For this review, take the finished solid that the model builds, in its own axes (mm). Face numbers are marked on the shaded views. A direction names the side the tool comes from. Give positions to 0.01 mm unless a question says otherwise; leave off trailing zeros. Order: outer loops, then holes, each group sorted by start corner. A loop starts at its lowest first (then second) coordinate and runs counter-clockwise, first axis right, second up. Notation, with made-up numbers: (-2, 23.25) -> (34, 23.25) arc R27 ccw to (34, 59.25) -> close; hole circle Ø6 at (66, 46). An arc over 180 degrees is marked (long way). Use CSV: the item, a comma, the result in double quotes. Start each with the question number.
Autodesk Inventor part; units mm, degrees
ref_plane "Work Plane1" through (12.15, 0, 0) normal (1, 0, 0) x (0, 0, -1)
ref_plane "YZ Plane" through (0, 0, 0) normal (1, 0, 0) x (0, 1, 0)
ref_plane "XZ Plane" through (0, 0, 0) normal (0, 1, 0) x (-1, 0, 0)
sketch "Sketch1" plane through (0, 0, 0) normal (1, 0, 0) x (0, 1, 0)
  line L0 (0, 0) -> (7.5, 0)
  line L1 (7.5, 0) -> (3.75, -6.4952)
  line L2 (3.75, -6.4952) -> (-3.75, -6.4952)
  line L3 (-3.75, -6.4952) -> (-7.5, 0)
  line L4 (-7.5, 0) -> (-3.75, 6.4952)
  line L5 (-3.75, 6.4952) -> (3.75, 6.4952)
  line L6 (3.75, 6.4952) -> (7.5, 0)
  circle A0 centre (0, 0) radius 15
  dimension "d0" = 7.5
  dimension "d1" = 30
extrude "Extrusion1" add sketch "Sketch1" along normal blind 10.25
sketch "Sketch2" plane through (10.25, 0, 0) normal (1, 0, 0) x (0, 0, -1)
  circle A0 centre (0, 0) radius 22.5
  line L0 (-6.4952, 3.75) -> (0, 7.5)
  line L1 (-6.4952, -3.75) -> (-6.4952, 3.75)
  line L2 (0, -7.5) -> (-6.4952, -3.75)
  line L3 (6.4952, -3.75) -> (0, -7.5)
  line L4 (6.4952, 3.75) -> (6.4952, -3.75)
  line L5 (0, 7.5) -> (6.4952, 3.75)
  dimension "d4" = 45
extrude "Extrusion2" add sketch "Sketch2" against normal blind 5
sketch "Sketch3" plane through (10.25, 0, 0) normal (1, 0, 0) x (0, 0, -1)
  circle A0 centre (0, 19.05) radius 1.45
  circle A1 centre (-16.4978, -9.525) radius 1.45
  circle A2 centre (16.4978, -9.525) radius 1.45
  point P0 (0, 0)
  dimension "d11" = 360
extrude "Extrusion3" cut sketch "Sketch3" against normal up to surface (5 mm away)
sketch "Sketch4" plane through (10.25, 0, 0) normal (1, 0, 0) x (0, 0, -1)
  circle A0 centre (0, 19.05) radius 1.45
  line L0 (-3, 17.2409) -> (-3, 16.225)
  line L1 (3, 17.2409) -> (3, 16.225)
  line L2 (13.3804, 11.279) -> (12.7273, 10.5007)
  line L3 (8.7841, 15.1357) -> (8.1311, 14.3574)
  line L4 (17.5, 0.0394) -> (16.4994, -0.137)
  line L5 (16.4581, 5.9483) -> (15.4575, 5.7719)
  line L6 (13.4311, -11.2185) -> (12.5512, -10.7106)
  line L7 (16.4311, -6.0224) -> (15.5512, -5.5144)
  arc A1 (8.7841, 15.1357) -> (3, 17.2409) centre (0, 0) ccw
  arc A2 (16.4311, -6.0224) -> (17.5, 0.0394) centre (0, 0) ccw
  arc A3 (16.4581, 5.9483) -> (13.3804, 11.279) centre (0, 0) ccw
  arc A4 (12.7273, 10.5007) -> (8.1311, 14.3574) centre (0, 0) ccw
  arc A5 (16.4994, -0.137) -> (15.4575, 5.7719) centre (0, 0) ccw
  line L8 (3.0777, -17.2272) -> (2.7302, -16.2726)
  line L9 (3.0777, -17.2272) -> (2.7302, -16.2726)
  line L10 (8.7158, -15.1751) -> (8.3683, -14.2204)
  line L11 (8.7158, -15.1751) -> (8.3683, -14.2204)
  line L12 (-8.7158, -15.1751) -> (-8.3683, -14.2204)
  line L13 (-8.7158, -15.1751) -> (-8.3683, -14.2204)
  line L14 (-3.0777, -17.2272) -> (-2.7302, -16.2726)
  line L15 (-3.0777, -17.2272) -> (-2.7302, -16.2726)
  line L16 (-16.4311, -6.0224) -> (-15.5512, -5.5144)
  line L17 (-16.4311, -6.0224) -> (-15.5512, -5.5144)
  line L18 (-13.4311, -11.2185) -> (-12.5512, -10.7106)
  line L19 (-13.4311, -11.2185) -> (-12.5512, -10.7106)
  arc A6 (8.7158, -15.1751) -> (13.4311, -11.2185) centre (0, 0) ccw
  arc A7 (-13.4311, -11.2185) -> (-8.7158, -15.1751) centre (0, 0) ccw
  arc A8 (-3.0777, -17.2272) -> (3.0777, -17.2272) centre (0, 0) ccw
  arc A9 (12.5512, -10.7106) -> (15.5512, -5.5144) centre (0, 0) ccw
  arc A10 (2.7302, -16.2726) -> (8.3683, -14.2204) centre (0, 0) ccw
  arc A11 (-8.3683, -14.2204) -> (-2.7302, -16.2726) centre (0, 0) ccw
  line L20 (-8.7841, 15.1357) -> (-8.1311, 14.3574)
  line L21 (-13.4115, 11.2412) -> (-12.7273, 10.5007)
  line L22 (-16.4586, 5.9455) -> (-15.4575, 5.7719)
  line L23 (-16.4311, -6.0224) -> (-15.5512, -5.5144)
  line L24 (-13.4311, -11.2185) -> (-12.5512, -10.7106)
  arc A12 (-3, 17.2409) -> (-8.7841, 15.1357) centre (0, 0) ccw
  arc A13 (-13.4115, 11.2412) -> (-15.8894, 7.3321) centre (0, 0) ccw
  arc A14 (-17.2328, -3.0466) -> (-16.4311, -6.0224) centre (0, 0) ccw
  arc A15 (-15.5512, -5.5144) -> (-12.5512, -10.7106) centre (0, 0) ccw
  arc A16 (3, 16.225) -> (-3, 16.225) centre (0, 0) ccw
  arc A17 (-8.1311, 14.3574) -> (-12.7273, 10.5007) centre (0, 0) ccw
  line L25 (-6.4952, 3.75) -> (0, 7.5)
  line L26 (-6.4952, -3.75) -> (-6.4952, 3.75)
  line L27 (0, -7.5) -> (-6.4952, -3.75)
  line L28 (6.4952, -3.75) -> (0, -7.5)
  line L29 (6.4952, 3.75) -> (6.4952, -3.75)
  line L30 (0, 7.5) -> (6.4952, 3.75)
  line L31 (-17.2328, -3.0466) -> (-16.181, -3.229)
  arc A18 (-3, 17.2409) -> (-8.7841, 15.1357) centre (0, 0) ccw
  arc A19 (8.7841, 15.1357) -> (3, 17.2409) centre (0, 0) ccw
  arc A20 (16.4581, 5.9483) -> (13.3804, 11.279) centre (0, 0) ccw
  arc A21 (16.4311, -6.0224) -> (17.5, 0.0394) centre (0, 0) ccw
  arc A22 (8.7158, -15.1751) -> (13.4311, -11.2185) centre (0, 0) ccw
  arc A23 (-3.0777, -17.2272) -> (3.0777, -17.2272) centre (0, 0) ccw
  arc A24 (-13.4311, -11.2185) -> (-8.7158, -15.1751) centre (0, 0) ccw
  arc A25 (-13.4115, 11.2412) -> (-16.4586, 5.9455) centre (0, 0) ccw
  arc A26 (3, 16.225) -> (-3, 16.225) centre (0, 0) ccw
  arc A27 (12.7273, 10.5007) -> (8.1311, 14.3574) centre (0, 0) ccw
  arc A28 (16.4994, -0.137) -> (15.4575, 5.7719) centre (0, 0) ccw
  arc A29 (12.5512, -10.7106) -> (15.5512, -5.5144) centre (0, 0) ccw
  arc A30 (2.7302, -16.2726) -> (8.3683, -14.2204) centre (0, 0) ccw
  arc A31 (-8.3683, -14.2204) -> (-2.7302, -16.2726) centre (0, 0) ccw
  arc A32 (-15.4575, 5.7719) -> (-16.181, -3.229) centre (0, 0) ccw
  arc A33 (-15.5512, -5.5144) -> (-12.5512, -10.7106) centre (0, 0) ccw
  arc A34 (-8.3683, -14.2204) -> (-2.7302, -16.2726) centre (0, 0) ccw
  arc A35 (2.7302, -16.2726) -> (8.3683, -14.2204) centre (0, 0) ccw
  arc A36 (12.5512, -10.7106) -> (15.5512, -5.5144) centre (0, 0) ccw
  arc A37 (16.4994, -0.137) -> (15.4575, 5.7719) centre (0, 0) ccw
  arc A38 (12.7273, 10.5007) -> (8.1311, 14.3574) centre (0, 0) ccw
  arc A39 (3, 16.225) -> (-3, 16.225) centre (0, 0) ccw
  arc A40 (-8.1311, 14.3574) -> (-12.7273, 10.5007) centre (0, 0) ccw
  line L32 (-16.181, -3.229) -> (-17.2328, -3.0466)
  line L33 (-8.7158, -15.1751) -> (-8.3683, -14.2204)
  line L34 (-3.0777, -17.2272) -> (-2.7302, -16.2726)
  line L35 (3.0777, -17.2272) -> (2.7302, -16.2726)
  line L36 (8.3683, -14.2204) -> (8.7158, -15.1751)
  line L37 (12.5512, -10.7106) -> (13.4311, -11.2185)
  line L38 (15.5512, -5.5144) -> (16.4311, -6.0224)
  line L39 (16.4994, -0.137) -> (17.5, 0.0394)
  line L40 (15.4575, 5.7719) -> (16.4581, 5.9483)
  line L41 (12.7273, 10.5007) -> (13.3804, 11.279)
  line L42 (8.1311, 14.3574) -> (8.7841, 15.1357)
  line L43 (3, 16.225) -> (3, 17.2409)
  line L44 (-3, 16.225) -> (-3, 17.2409)
  line L45 (-8.1311, 14.3574) -> (-8.7841, 15.1357)
  line L46 (-12.7273, 10.5007) -> (-13.3804, 11.279)
  line L47 (-12.7273, 10.5007) -> (-13.3804, 11.279)
  line L48 (-15.4575, 5.7719) -> (-16.4586, 5.9455)
  line L49 (-16.181, -3.229) -> (-17.2328, -3.0466)
  line L50 (-16.4311, -6.0224) -> (-15.5512, -5.5144)
  line L51 (-13.4311, -11.2185) -> (-12.5512, -10.7106)
  line L52 (-8.7158, -15.1751) -> (-8.3683, -14.2204)
  line L53 (-3.0777, -17.2272) -> (-2.7302, -16.2726)
  line L54 (3.0777, -17.2272) -> (2.7302, -16.2726)
  point P0 (15.5512, -5.5144)
  point P1 (-8.7158, -15.1751)
  point P2 (-3.0777, -17.2272)
  point P3 (3.0777, -17.2272)
  point P4 (2.7302, -16.2726)
  point P5 (8.7158, -15.1751)
  point P6 (-15.5512, -5.5144)
  point P7 (-2.7302, -16.2726)
  point P8 (-8.3683, -14.2204)
  point P9 (8.3683, -14.2204)
  point P10 (2.7302, -16.2726)
ref_plane "Work Plane1" through (12.15, 0, 0) normal (1, 0, 0) x (0, 0, -1)
sketch "Sketch5" plane through (12.15, 0, 0) normal (1, 0, 0) x (0, 0, -1)
  line L0 (6.4952, 3.75) -> (6.4952, -3.75)
  circle A0 centre (0, 0) radius 7.5
extrude "Extrusion6" add sketch "Sketch4" along normal blind 2 contours L0 A16 L1 A1 L3 A4 L2 A3 L5 A5 L4 A2 L7 A9 L6 A6 L10 A10 L8 A8 L14 A11 L12 A7 L18 A15 L16 A14 L31 A32 L22 A25 A13 L21 A17 L20 A12
sketch "Sketch6" plane through (12.25, 0, 0) normal (1, 0, 0) x (0, 0, -1)
  arc A0 (-13.4115, 11.2412) -> (-16.4586, 5.9455) centre (0, 0) ccw
  line L0 (-16.4586, 5.9455) -> (-15.4575, 5.7719)
  arc A1 (-15.4575, 5.7719) -> (-16.181, -3.229) centre (0, 0) ccw
  line L1 (-16.181, -3.229) -> (-17.2328, -3.0466)
  arc A2 (-17.2328, -3.0466) -> (-16.4311, -6.0224) centre (0, 0) ccw
  line L2 (-16.4311, -6.0224) -> (-15.5512, -5.5144)
  arc A3 (-15.5512, -5.5144) -> (-12.5512, -10.7106) centre (0, 0) ccw
  line L3 (-12.5512, -10.7106) -> (-13.4311, -11.2185)
  arc A4 (-13.4311, -11.2185) -> (-8.7158, -15.1751) centre (0, 0) ccw
  line L4 (-8.7158, -15.1751) -> (-8.3683, -14.2204)
  arc A5 (-8.3683, -14.2204) -> (-2.7302, -16.2726) centre (0, 0) ccw
  line L5 (-2.7302, -16.2726) -> (-3.0777, -17.2272)
  arc A6 (-3.0777, -17.2272) -> (3.0777, -17.2272) centre (0, 0) ccw
  line L6 (3.0777, -17.2272) -> (2.7302, -16.2726)
  arc A7 (2.7302, -16.2726) -> (8.3683, -14.2204) centre (0, 0) ccw
  line L7 (8.3683, -14.2204) -> (8.7158, -15.1751)
  arc A8 (8.7158, -15.1751) -> (13.4311, -11.2185) centre (0, 0) ccw
  line L8 (13.4311, -11.2185) -> (12.5512, -10.7106)
  arc A9 (12.5512, -10.7106) -> (15.5512, -5.5144) centre (0, 0) ccw
  line L9 (15.5512, -5.5144) -> (16.4311, -6.0224)
  arc A10 (16.4311, -6.0224) -> (17.5, 0.0394) centre (0, 0) ccw
  line L10 (17.5, 0.0394) -> (16.4994, -0.137)
  arc A11 (16.4994, -0.137) -> (15.4575, 5.7719) centre (0, 0) ccw
  line L11 (15.4575, 5.7719) -> (16.4581, 5.9483)
  arc A12 (16.4581, 5.9483) -> (13.3804, 11.279) centre (0, 0) ccw
  line L12 (13.3804, 11.279) -> (12.7273, 10.5007)
  arc A13 (12.7273, 10.5007) -> (8.1311, 14.3574) centre (0, 0) ccw
  line L13 (8.1311, 14.3574) -> (8.7841, 15.1357)
  arc A14 (8.7841, 15.1357) -> (3, 17.2409) centre (0, 0) ccw
  line L14 (3, 17.2409) -> (3, 16.225)
  arc A15 (3, 16.225) -> (-3, 16.225) centre (0, 0) ccw
  line L15 (-3, 16.225) -> (-3, 17.2409)
  arc A16 (-3, 17.2409) -> (-8.7841, 15.1357) centre (0, 0) ccw
  line L16 (-8.7841, 15.1357) -> (-8.1311, 14.3574)
  arc A17 (-8.1311, 14.3574) -> (-12.7273, 10.5007) centre (0, 0) ccw
  line L17 (-12.7273, 10.5007) -> (-13.4115, 11.2412)
  line L18 (-6.4952, 3.75) -> (0, 7.5)
  line L19 (0, 7.5) -> (6.4952, 3.75)
  line L20 (6.4952, 3.75) -> (6.4952, -3.75)
  line L21 (6.4952, -3.75) -> (0, -7.5)
  line L22 (0, -7.5) -> (-6.4952, -3.75)
  line L23 (-6.4952, -3.75) -> (-6.4952, 3.75)
  arc A18 (3, 16.225) -> (-3, 16.225) centre (0, 0) ccw
  line L24 (3, 16.225) -> (3, 15.9707)
  line L25 (8.1311, 14.3574) -> (7.9676, 14.1626)
  line L26 (12.7273, 10.5007) -> (12.5639, 10.3059)
  line L27 (15.4575, 5.7719) -> (15.2071, 5.7277)
  line L28 (16.4994, -0.137) -> (16.249, -0.1811)
  line L29 (15.5512, -5.5144) -> (16.4311, -6.0224)
  line L30 (15.5512, -5.5144) -> (15.331, -5.3873)
  line L31 (12.5512, -10.7106) -> (13.4311, -11.2185)
  line L32 (12.5512, -10.7106) -> (12.331, -10.5834)
  line L33 (8.7158, -15.1751) -> (8.3683, -14.2204)
  line L34 (8.3683, -14.2204) -> (8.2814, -13.9815)
  line L35 (2.7302, -16.2726) -> (2.6432, -16.0336)
  arc A19 (-8.3683, -14.2204) -> (-2.7302, -16.2726) centre (0, 0) ccw
  line L36 (-2.7302, -16.2726) -> (-2.6432, -16.0336)
  line L37 (-8.3683, -14.2204) -> (-8.2814, -13.9815)
  line L38 (-12.5512, -10.7106) -> (-12.331, -10.5834)
  line L39 (-15.5512, -5.5144) -> (-15.331, -5.3873)
  arc A20 (-15.4575, 5.7719) -> (-16.181, -3.229) centre (0, 0) ccw
  line L40 (-16.181, -3.229) -> (-15.9166, -3.2749)
  line L41 (-15.4575, 5.7719) -> (-15.2068, 5.7284)
  line L42 (-12.7273, 10.5007) -> (-12.5561, 10.3154)
  line L43 (-8.1311, 14.3574) -> (-7.9676, 14.1626)
  line L44 (-3, 16.225) -> (-3, 15.9707)
  arc A21 (-7.9676, 14.1626) -> (-12.5561, 10.3154) centre (0, 0) ccw
  arc A22 (-15.2068, 5.7284) -> (-15.9166, -3.2749) centre (0, 0) ccw
  arc A23 (-15.331, -5.3873) -> (-12.331, -10.5834) centre (0, 0) ccw
  arc A24 (-8.2814, -13.9815) -> (-2.6432, -16.0336) centre (0, 0) ccw
  arc A25 (2.6432, -16.0336) -> (8.2814, -13.9815) centre (0, 0) ccw
  arc A26 (12.331, -10.5834) -> (15.331, -5.3873) centre (0, 0) ccw
  arc A27 (16.249, -0.1811) -> (15.2071, 5.7277) centre (0, 0) ccw
  arc A28 (12.5639, 10.3059) -> (7.9676, 14.1626) centre (0, 0) ccw
  arc A29 (3, 15.9707) -> (-3, 15.9707) centre (0, 0) ccw
  arc A30 (-3, 16.9871) -> (-8.621, 14.9413) centre (0, 0) ccw
  arc A31 (-13.2408, 11.0564) -> (-16.2089, 5.9022) centre (0, 0) ccw
  arc A32 (-16.9706, -3.092) -> (-16.2113, -5.8955) centre (0, 0) ccw
  arc A33 (-13.2113, -11.0916) -> (-8.629, -14.9366) centre (0, 0) ccw
  arc A34 (-2.9909, -16.9887) -> (2.9909, -16.9887) centre (0, 0) ccw
  arc A35 (8.629, -14.9366) -> (13.2113, -11.0916) centre (0, 0) ccw
  arc A36 (16.2113, -5.8955) -> (17.25, -0.0046) centre (0, 0) ccw
  arc A37 (16.2081, 5.9042) -> (13.2172, 11.0845) centre (0, 0) ccw
  arc A38 (8.621, 14.9413) -> (3, 16.9871) centre (0, 0) ccw
  circle A39 centre (0, 0) radius 17.5
  point P0 (-8.7158, -15.1751)
  point P1 (3.0777, -17.2272)
  point P2 (13.4311, -11.2185)
  point P3 (17.5, 0.0394)
  point P4 (3, 17.2409)
  point P5 (-16.4311, -6.0224)
  point P6 (16.2113, -5.8955)
  point P7 (13.2113, -11.0916)
  point P8 (8.629, -14.9366)
extrude "Extrusion7" cut sketch "Sketch6" against normal up to surface (2 mm away) contours L17 A31 L0 A0 | A39 L16 A17 L17 | L0 A1 L1 A39 | A16 L15 A30 L16 | L1 A32 L2 A2 | A17 L43 A21 L42 | A39 L14 A15 L15 | L41 A22 L40 A1 | L2 A3 L3 A39 | A14 L13 A38 L14 | L3 A33 L4 A4 | A15 L24 A29 L44 | A39 L12 A13 L13 | L39 A23 L38 A3 | L4 A5 L5 A39 | A12 L11 A37 L12 | L5 A34 L6 A6 | A13 L26 A28 L25 | A39 L10 A11 L11 | L37 A24 L36 A5 | L6 A7 L7 A39 | A10 L9 A36 L10 | L7 A35 L8 A8 | A11 L28 A27 L27 | L35 A25 L34 A7 | L8 A9 L9 A39 | A9 L32 A26 L30
properties part number "wheel_gearing_mount_short"
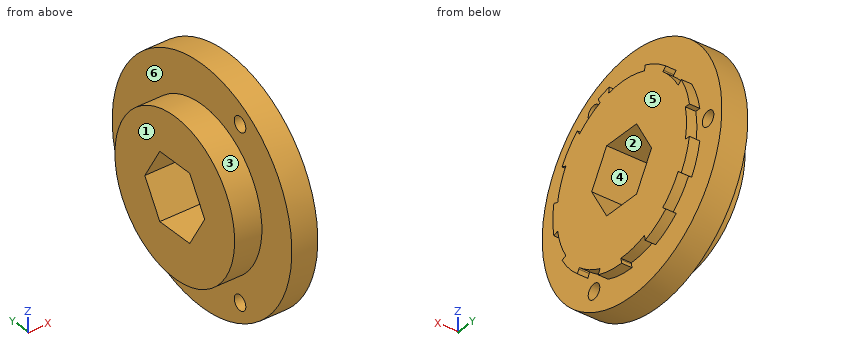
1. Consider section A-A (y = 19.05). State the section outline as (x, z) points, plus the area to 3 significant figures.
2. Clearance check with flat-ended pins moving along their axes: P1, Ø1, axis at x = 4, z = -11.5, coming from the -Y side; P2, Ø1.5, axis at y = -7, z = 16, coming from the +X side; P3, Ø4, axis at y = 19.05, z = 0, coming from the -X side; P4, Ø22.5, axis at y = 9, z = -10, coming from the -X side. State where each tip first meets the part, or that it passes through.
3. Consider section D-D (y = -18). State the section outline as (x, z) points.
4. Draft analysis for pull direction Y (two halves, no side actions). For the marked faces 1, 2 and 3, state which applies: +Y half, -Y half, draft (parallel to the pull), parting line (faces both ways), or undercut.
5. To check wall thickness, follow L1, parallel to Y at x = 7.2, z = 0; L2, parallel to X at y = -21, z = -2; L3, parallel to Y at x = 6.5, z = 3. State the ranges of each line that lie inside material, in increasing order. Write a range as [from, to].
6. Consider section B-B (z = -11.5). State the section outline as (x, y) points.
7. For the marked faces 4, 5 and 6, list the 3-axis set-ups (+Z, -Z, +X, -X, +Y, -Y) from which the entire face can be reached by the end or side of a thin tool; tool diameter is ignored.
8. Consider section C-C (y = 2). State the section outline as (x, z) points.
Answer list:
1,outline,"(5.25, -11.97) -> (10.25, -11.97) -> (10.25, -1.45) -> (5.25, -1.45) -> close; (5.25, 1.45) -> (10.25, 1.45) -> (10.25, 11.97) -> (5.25, 11.97) -> close"
1,area,"105 mm2"
2,P1,"y = -10.2"
2,P2,"x = 10.25"
2,P3,"x = 5.25"
2,P4,"x = 0"
3,outline,"(5.25, -13.5) -> (10.25, -13.5) -> (10.25, 13.5) -> (5.25, 13.5) -> close"
4,face 1,"draft"
4,face 2,"undercut"
4,face 3,"parting line"
5,L1,"[-22.5, -7.5], [7.5, 17.6], [20.5, 22.5]"
5,L2,"[5.25, 10.25]"
5,L3,"[-22.3, -5.77], [5.77, 22.3]"
6,outline,"(0, -9.63) -> (5.25, -9.63) -> (5.25, -19.34) -> (10.25, -19.34) -> (10.25, -12.86) -> (12.25, -12.86) -> (12.25, 11.48) -> (10.25, 11.48) -> (10.25, 19.34) -> (5.25, 19.34) -> (5.25, 9.63) -> (0, 9.63) -> close"
7,face 4,"+X, -X"
7,face 5,"+Z, -Z, +X, +Y, -Y"
7,face 6,"-X"
8,outline,"(0, -14.87) -> (5.25, -14.87) -> (5.25, -22.41) -> (10.25, -22.41) -> (10.25, -16.13) -> (12.25, -16.13) -> (12.25, -6.5) -> (0, -6.5) -> close; (0, 6.5) -> (12.25, 6.5) -> (12.25, 16.13) -> (10.25, 16.13) -> (10.25, 22.41) -> (5.25, 22.41) -> (5.25, 14.87) -> (0, 14.87) -> close"
